```python
from build123d import *

# Parameters (mm, degrees)
F0_W     = 160.02
F0_H     = 71.12
F1_DEPTH = 254
F2_W     = 38.1
F2_H     = 30.48
F2_W_2   = 38.099997
F2_W_3   = 35.56
F2_H_2   = 55.88
F3_DEPTH = 12.7
F5_W     = 38.1
F5_H     = 30.48
F6_DEPTH = 12.7
F7_R     = 5.08


with BuildPart() as f1:
    # F0 (on Front) → F1 (new body)
    with BuildSketch(Plane.XZ):
        with Locations((-1.466153, -28.354255)):
            Rectangle(F0_W, F0_H)
        Polygon((-88.9, 7.205745), (-81.476153, 7.205745), (78.543847, 7.205745), (88.9, 7.205745), (0, 56.392634), align=None)
    extrude(amount=F1_DEPTH)

    # F2 (on face) → F3 (cut)
    with BuildSketch(Plane.YZ.offset(78.543847)):
        with Locations((-200.764716, -23.274255)):
            Rectangle(F2_W, F2_H)
        with Locations((-51.652463, -23.274255)):
            Rectangle(F2_W_2, F2_H)
        with Locations((-125.025785, -35.974255)):
            Rectangle(F2_W_3, F2_H_2)
    extrude(amount=-F3_DEPTH, mode=Mode.SUBTRACT)

    # F5 (on face) → F6 (cut)
    with BuildSketch(Plane(origin=(-81.476153, 0, 0), x_dir=(0, -1, 0), z_dir=(-1, 0, 0))):
        with Locations((35.715754, -23.274255)):
            Rectangle(F5_W, F5_H)
        with Locations((129.347243, -23.274255)):
            Rectangle(F5_W, F5_H)
        with Locations((217.621587, -23.274255)):
            Rectangle(F5_W, F5_H)
    extrude(amount=-F6_DEPTH, mode=Mode.SUBTRACT)

    # F7
    f7_edges = [f1.edges().sort_by_distance(p)[0] for p in [
        (0, -127, 56.392634),
    ]]
    fillet(f7_edges, radius=F7_R)


solid = f1.part
```
Input: part model. Units: mm. Frame: model coordinates. A direction names the side the tool comes from. Coordinates: 2 decimals unless noted, no trailing zeros. Loops run counter-clockwise (first coordinate to the right, second up) from the corner with the lowest first, then second, coordinate; pieces in that order, holes last. Notation, with made-up numbers: M -9,10.25 L 5,10.25 A20 ccw 5,26.25 Z; hole C 65.5,63.5 d6. An arc over 180 degrees is marked long. Use a Markdown table: item, result. Add a question column.
1) Section D-D, the plane x = 39. Return the cut outline in (y, z).
2) Section C-C, the plane y = -67. Return the cut outline in (x, z), plus the area to 3 significant figures.
3) Section B-B, the plane y = -135.5. Return the cut outline in (x, z), plus the area to 3 significant figures.
4) Draft query along Z for faces 5 (the flat face through (-75, -35, -38.514)), 6 (the flat face through (84, -125, 7.206)), 7 (the flat face through (72, -142.806, -36)). Return one class per face: +Z half, -Z half, draft (parallel to the pull), parting line (faces both ways), or undercut.
5) Section A-A, the plane z = -47. Return the cut outline in (x, y), plus the area to 3 significant figures.
6) Set-up query: faces 1 (the flat face through (-75, -35, -8.034)), 2 (the flat face through (-3, -125, -63.914)), 3 (the flat face through (-81.476, -125, -45)), 4 (the flat face through (72, -201, -38.514)). Return all of +Z, -Z, +X, -X, +Y, -Y with unobstructed straight access to the full face (end or side cutting, diameter ignored); none if empty.
7) Pin query (flat end, axial travel): P1, Ø10, axis at y = -200, z = 15.5, coming from the +X side; P2, Ø12, axis at y = -165.5, z = 41.5, coming from the +X side; P3, Ø5, axis at x = 84.5, y = -103, coming from the -Z side. Return the tip coordinate at first contact, or that it passes through.
8) Line query: L1, parallel to Y at x = 69, z = -13.5; L2, parallel to X at y = -221.5, z = -25; L3, parallel to Y at x = 74.5, z = -45. Output: solid intervals per line, ascending. Write a range as from..to.
Answer below:
| question | item | result |
|---|---|---|
| 1 | outline | M -254,-63.91 L 0,-63.91 L 0,34.81 L -254,34.81 Z |
| 2 | outline | M -88.9,7.21 L -81.48,7.21 L -81.48,-63.91 L 78.54,-63.91 L 78.54,-38.51 L 65.84,-38.51 L 65.84,-8.03 L 78.54,-8.03 L 78.54,7.21 L 88.9,7.21 L 2.46,55.03 A5.08 ccw -2.46,55.03 Z |
| 2 | area | 15,400 mm2 |
| 3 | outline | M -88.9,7.21 L -81.48,7.21 L -81.48,-8.03 L -68.78,-8.03 L -68.78,-38.51 L -81.48,-38.51 L -81.48,-63.91 L 65.84,-63.91 L 65.84,-8.03 L 78.54,-8.03 L 78.54,7.21 L 88.9,7.21 L 2.46,55.03 A5.08 ccw -2.46,55.03 Z |
| 3 | area | 14,700 mm2 |
| 4 | face 5 | undercut |
| 4 | face 6 | -Z half |
| 4 | face 7 | draft |
| 5 | outline | M -81.48,-254 L 78.54,-254 L 78.54,-142.81 L 65.84,-142.81 L 65.84,-107.25 L 78.54,-107.25 L 78.54,0 L -81.48,0 Z |
| 5 | area | 40,200 mm2 |
| 6 | face 1 | -X |
| 6 | face 2 | -Z, +X, -X, +Y, -Y |
| 6 | face 3 | -Z, -X, +Y, -Y |
| 6 | face 4 | +X |
| 7 | P1 | x = 82.95 |
| 7 | P2 | x = 37.76 |
| 7 | P3 | z = 7.21 |
| 8 | L1 | -254..-219.81, -181.71..-142.81, -107.25..-70.7, -32.6..0 |
| 8 | L2 | -68.78..78.54 |
| 8 | L3 | -254..-142.81, -107.25..0 |
